from build123d import *

# Parameters (mm, degrees)
F0_W     = 152.4
F0_H     = 114.3
F1_DEPTH = 12.7
F3_DEPTH = 38.1


with BuildPart() as f1:
    # F0 (on Front) → F1 (new body)
    with BuildSketch(Plane.XZ):
        Rectangle(F0_W, F0_H)
    extrude(amount=F1_DEPTH)

    # F2 (on face) → F3 (join)
    with BuildSketch(Plane(origin=(0, 0, 0), x_dir=(-1, 0, 0), z_dir=(0, 1, 0))):
        with BuildLine():
            Line((-42.303127, 15.852345), (2.400873, -17.675655))
            ThreePointArc((2.400873, -17.675655), (20.180873, -15.135655), (17.640873, 2.644345))
            Line((17.640873, 2.644345), (-27.063127, 36.172345))
            ThreePointArc((-27.063127, 36.172345), (-44.843127, 33.632345), (-42.303127, 15.852345))
        make_face()
    extrude(amount=F3_DEPTH)


solid = f1.part
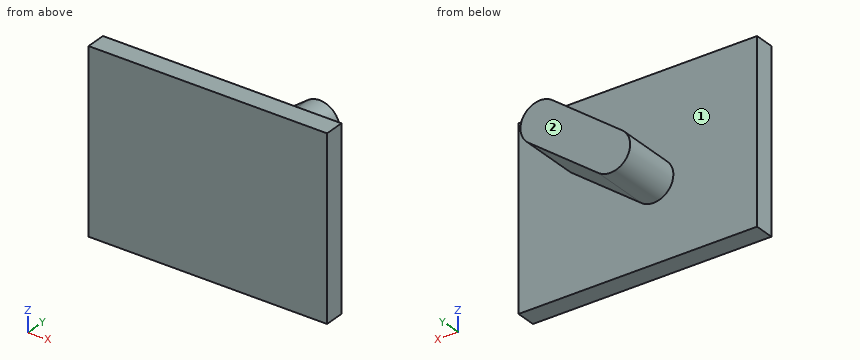
Input: part model. Units: mm. Frame: model coordinates. Face numbers are marked on the shaded views. A direction names the side the tool comes from. Coordinates: 2 decimals unless noted, no trailing zeros. Write each loop counter-clockwise with the first axis right and the second up, starting at its lowest first coordinate (ties: lowest second). Pieces come first, ordered by that corner, then holes. Notation, with made-up numbers: M 79.5,25 L 96.5,25 A26 cw 96.5,50 Z; hole C -28.75,23 d9. An arc over 180 degrees is marked long. Answer as a JSON object with one key per item and string values. Group by question number.
(1) Ray query, line 1 along Y through (x, z) = (-32.5, 15.5); line 2 along Z through (x, y) = (-6, 8.5) (3 decimals); line 3 along X through (y, z) = (31, 1.5). Return the intervals inside material, ascending. Write a range as [from, to].
(2) Section B-B on y = 14.5. Output: boundary loops of the cut face in (x, z).
(3) Section C-C on x = -42. Output: boundary loops of the cut face in (y, z), plus the area to 3 significant figures.
(4) Set-up query: the marked faces 1 and 2. Return all of +Z, -Z, +X, -X, +Y, -Y with unobstructed straight access to the full face (end or side cutting, diameter ignored); none if empty.
(5) Section A-A on z = 7. Output: boundary loops of the cut face in (x, y), plus the area to 3 significant figures.
(6) Section D-D on z = -13.5. Output: boundary loops of the cut face in (x, y), plus the area to 3 significant figures.
(7) Contact query for flat-ended pins moving along their axis: P1, Ø10, axis at x = 0.5, z = 32.5, coming from the +Y side; P2, Ø4, axis at x = 13, y = 23.5, coming from the -Z side (3 decimals); P3, Ø6, axis at x = -24.5, y = 10.5, coming from the +Z side. Output: stop coordinate, or through.
Result set:
{
 "1": {"line 1": "y = [-12.7, 0]", "line 2": "z = [-19.562, 11.375]", "line 3": "x = [-18.97, 23.17]"},
 "2": {"outline": "M -17.64,2.64 A12.7 ccw -2.4,-17.68 L 42.3,15.85 A12.7 ccw 27.06,36.17 Z"},
 "3": {"outline": "M -12.7,-57.15 L 0,-57.15 L 0,57.15 L -12.7,57.15 Z", "area": "1,450 mm2"},
 "4": {"face 1": "+Y", "face 2": "+Z, -Z, +X, -X, +Y"},
 "5": {"outline": "M -76.2,-12.7 L 76.2,-12.7 L 76.2,0 L 30.5,0 L 30.5,38.1 L -11.83,38.1 L -11.83,0 L -76.2,0 Z", "area": "3,550 mm2"},
 "6": {"outline": "M -76.2,-12.7 L 76.2,-12.7 L 76.2,0 L 3.17,0 L 3.17,38.1 L -21.22,38.1 L -21.22,0 L -76.2,0 Z", "area": "2,860 mm2"},
 "7": {"P1": "stops at y = 0", "P2": "stops at z = -7.625", "P3": "stops at z = -2.08"}
}
